from build123d import *

# Parameters (mm, degrees)
SKETCH2_R           = 2.0828
BOSS_EXTRUDE1_DEPTH = 6.35


with BuildPart() as part:
    # Sketch2 → Boss-Extrude1 (new body)
    with BuildSketch(Plane(origin=(0, 0, 0), x_dir=(1, 0, 0), z_dir=(0, 1, 0))):
        Polygon((3.175, 0), (3.175, 12.7), (-3.175, 12.7), (-3.175, 25.4), (3.175, 25.4), (3.175, 38.1), (-3.175, 38.1), (-3.175, 50.8), (3.175, 50.8), (3.175, 63.5), (-3.175, 63.5), (-3.175, 76.2), (3.175, 76.2), (3.175, 88.9), (-3.175, 88.9), (-3.175, 101.6), (3.175, 101.6), (3.175, 114.3), (-3.175, 114.3), (-3.175, 127), (3.175, 127), (142.875, 127), (149.225, 127), (149.225, 114.3), (142.875, 114.3), (142.875, 101.6), (149.225, 101.6), (149.225, 88.9), (142.875, 88.9), (142.875, 76.2), (149.225, 76.2), (149.225, 63.5), (142.875, 63.5), (142.875, 50.8), (149.225, 50.8), (149.225, 38.1), (142.875, 38.1), (142.875, 25.4), (149.225, 25.4), (149.225, 12.7), (142.875, 12.7), (142.875, 0), align=None)
        with Locations(Location((136.525, 57.15, 0), (0, 0, 90))):
            Circle(SKETCH2_R, mode=Mode.SUBTRACT)
        with Locations(Location((9.525, 12.7, 0), (0, 0, 270))):
            Circle(SKETCH2_R, mode=Mode.SUBTRACT)
        with Locations(Location((9.525, 57.15, 0), (0, 0, 270))):
            Circle(SKETCH2_R, mode=Mode.SUBTRACT)
        with Locations(Location((136.525, 12.7, 0), (0, 0, 90))):
            Circle(SKETCH2_R, mode=Mode.SUBTRACT)
    extrude(amount=BOSS_EXTRUDE1_DEPTH)


solid = part.part
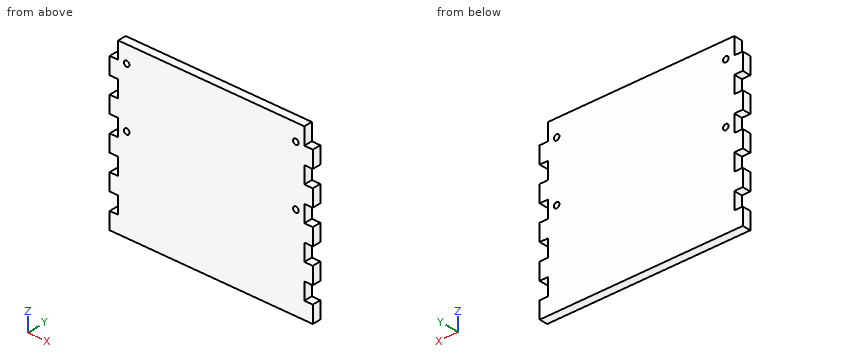
Part model, mm, in its own coordinate system. Coordinates: 2 decimals unless noted, no trailing zeros. Order: outer loops, then holes, each group sorted by start corner. A loop starts at its lowest first (then second) coordinate and runs counter-clockwise, first axis right, second up. Notation, with made-up numbers: M 36,64 L 93,64 A26 cw 93,101 Z; hole C -10.5,-23 d2. An arc over 180 degrees is marked long. Use a Markdown table: item, result.
(1) Cut at B-B on y = 2.25. State how many separate pieces and enclosed holes the cut face has, then the cut area to 3 significant figures.
A:
| item | result |
|---|---|
| separate pieces | 1 |
| enclosed holes | 4 |
| area | 18,500 mm^2 |
(2) Cut at A-A on z = -57.15. Write the cut outline in (x, y) (3 decimals).
A:
| item | result |
|---|---|
| outline | M 3.175,0 L 7.442,0 L 7.442,6.35 L 3.175,6.35 Z; M 11.608,0 L 134.442,0 L 134.442,6.35 L 11.608,6.35 Z; M 138.608,0 L 142.875,0 L 142.875,6.35 L 138.608,6.35 Z |
(3) Probe L1, parallel to X at y = 1.5, z = -57.15 (3 decimals); L2, parallel to Z at x = 8, y = 2.5; L3, parallel to X at y = 0.5, z = -26 (3 decimals). List the from-to ranges inside material, lowest first.
A:
| item | result |
|---|---|
| L1 | x = 3.175 to 7.442, 11.608 to 134.442, 138.608 to 142.875 |
| L2 | z = -127 to -58.57, -55.73 to -14.12, -11.28 to 0 |
| L3 | x = 3.175 to 142.875 |
(4) Flat gauge pins, fed straight in: pin 1 (1.9 mm diameter, centred on x = 147, y = 1.5, fed in from +Z); pin 2 (3 mm diameter, centred on y = 2, z = -82, fed in from -X) (3 decimals). Where does each tip first touch, or does it go through?
A:
| item | result |
|---|---|
| pin 1 | stops at z = -12.7 |
| pin 2 | stops at x = 3.175 |
